For this review, use the dimensioned drawing (mm, ordinates from the lowest corner) and the shaded views. A direction names the side the tool comes from. Give positions to 0.01 mm unless a question says otherwise; leave off trailing zeros. Write each loop counter-clockwise with the first axis right and the second up, starting at its lowest first coordinate (ties: lowest second). Pieces come first, ordered by that corner, then holes. Notation, with made-up numbers: M -23,-12.75 L 5,-12.75 A23 ccw 5,-4.75 Z; hole C 14.25,32 d2. An arc over 180 degrees is marked long. Answer in a Markdown table with one row per item.
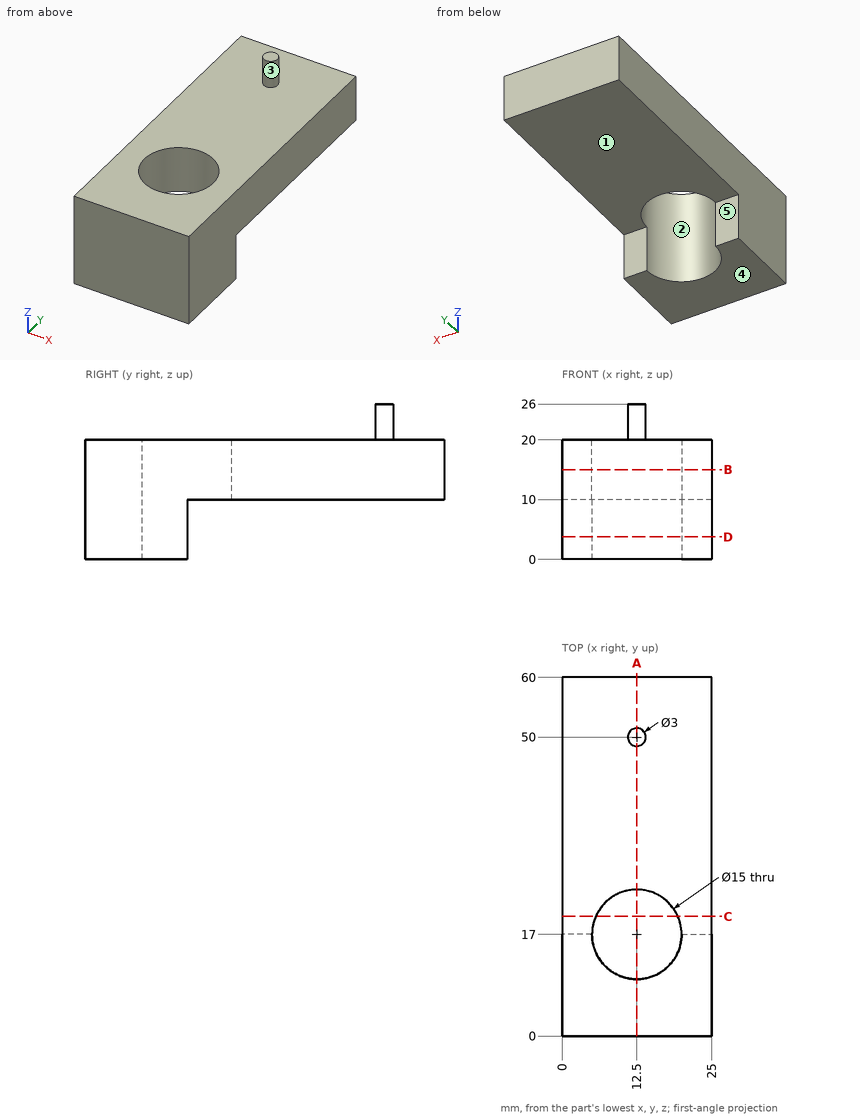
1) Add section D-D (z = 3.75). Write out the cut boundary in (x, y), and give its area (3 significant figures).
Geometry says:
| item | result |
|---|---|
| outline | M 0,0 L 25,0 L 25,17 L 20,17 A7.5 cw 5,17 L 0,17 Z |
| area | 337 mm^2 |
2) Insertion check: P1, Ø5.5, axis at x = 3, z = 4, coming from the +Y side; P2, Ø9, axis at x = 12.5, y = 17, coming from the +Z side; P3, Ø12, axis at y = 47.5, z = 20.5, coming from the +X side; P4, Ø8, axis at x = 13, y = 31.5, coming from the -Z side. Each pin has a flat end and moves straight along its axis. Give the tip position at first contact, or say it passes through.
Geometry says:
| item | result |
|---|---|
| P1 | y = 17 |
| P2 | through |
| P3 | x = 25 |
| P4 | z = 10 |
3) Add section B-B (z = 15). Write out the cut boundary in (x, y), and give its area (3 significant figures).
Geometry says:
| item | result |
|---|---|
| outline | M 0,0 L 25,0 L 25,60 L 0,60 Z; hole C 12.5,17 d15 |
| area | 1,320 mm^2 |
4) Add section A-A (x = 12.5). Write out the cut boundary in (y, z), and give its area (3 significant figures).
Geometry says:
| item | result |
|---|---|
| outline | M 0,0 L 9.5,0 L 9.5,20 L 0,20 Z; M 24.5,10 L 60,10 L 60,20 L 51.5,20 L 51.5,26 L 48.5,26 L 48.5,20 L 24.5,20 Z |
| area | 563 mm^2 |
5) For the marked faces 4 and 5, list the 3-axis set-ups (+Z, -Z, +X, -X, +Y, -Y) from which the entire face can be reached by the end or side of a thin tool; tool diameter is ignored.
Geometry says:
| item | result |
|---|---|
| face 4 | -Z, +X, -X, +Y, -Y |
| face 5 | -Z, +X, -X, +Y |
6) Add section C-C (y = 20). Write out the cut boundary in (x, z), and give its area (3 significant figures).
Geometry says:
| item | result |
|---|---|
| outline | M 0,10 L 5.63,10 L 5.63,20 L 0,20 Z; M 19.37,10 L 25,10 L 25,20 L 19.37,20 Z |
| area | 113 mm^2 |
7) To check wall thickness, follow probe 1 along X at (y, z) = (17, 11.5); probe 2 along Y at (x, z) = (12.5, 10.5); probe 3 along Z at (x, y) = (17.75, 52). State the ranges of each line that lie inside material, in increasing order. Write a range as [from, to].
Geometry says:
| item | result |
|---|---|
| probe 1 | [0, 5], [20, 25] |
| probe 2 | [0, 9.5], [24.5, 60] |
| probe 3 | [10, 20] |
8) The part is to be moulded in two halves that separate along X. For the marked faces 1, 2 and 3, say which applies: released by +X, released by -X, zero draft, split by the parting line, or undercut.
Geometry says:
| item | result |
|---|---|
| face 1 | zero draft |
| face 2 | undercut |
| face 3 | split by the parting line |
